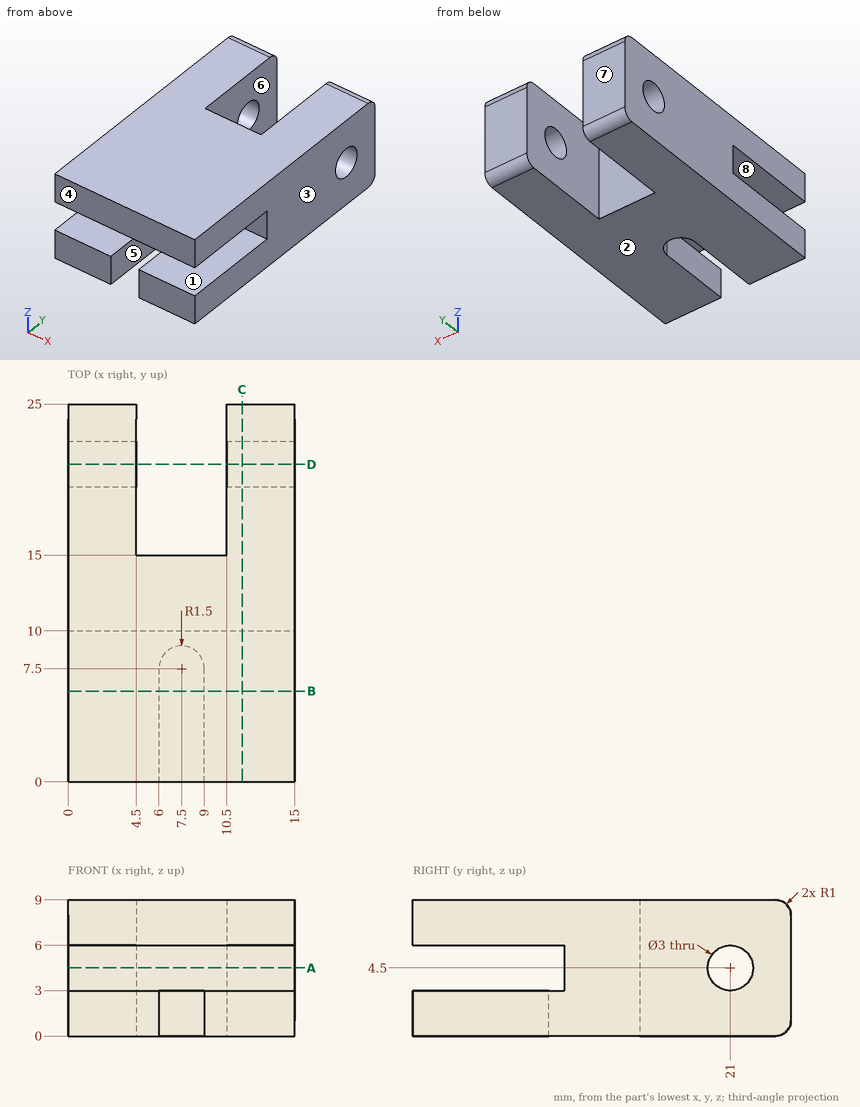
Geometry: see drawing. Coordinates: mm, zero at the bounding-box minimum. A direction names the side the tool comes from. Coordinates: 2 decimals unless noted, no trailing zeros. Loops run counter-clockwise (first coordinate to the right, second up) from the corner with the lowest first, then second, coordinate; pieces in that order, holes last. Notation, with made-up numbers: M 46.25,-35 L 103.25,-35 A31 ccw 103.25,-6 Z; hole C 18,30 d10. An arc over 180 degrees is marked long. Put each result on its own line as item: value. Start each with the question number.
1) Reachability of the marked faces 4, 5, 6, 7 and 8 from +Z, -Z, +X, -X, +Y, -Y: full face, straight path, thin tool, end or side. Return the list, or none.
2) Contact query for a flat-ended pin moving along its axis: pin 1 Ø2.5 at (x, z) = (10, 4.5) entering from -Y. Output: stop coordinate, or through.
3) Ray query, L1, parallel to X at y = 22, z = 8.25; L2, parallel to Y at x = 3.25, z = 4.5; L3, parallel to Z at x = 12.7, y = 21. Return the intervals inside material, ascending. Write a range as from..to.
4) Cut plane A-A on z = 4.5. Return the cut outline in (x, y), then the cut area to 3 significant figures.
5) Cut plane D-D on y = 21. Return the cut outline in (x, z), then the cut area to 3 significant figures.
6) Cut plane C-C on x = 11.5. Return the cut outline in (y, z), then the cut area to 3 significant figures.
7) Pull-direction query (Z, two-part tool) for the marked faces 1, 2 and 3; classes: pulls with the +Z half, pulls with the -Z half, needs draft (parallel to the pull), parting line crosses it, or undercut.
8) Cut plane B-B on y = 6. Return the cut outline in (x, z).
The answers:
1. face 4: +Z, -Z, +X, -X, -Y
1. face 5: -Z, -Y
1. face 6: +Z, -Z, +Y
1. face 7: +Z, -Z, +X, -X, +Y
1. face 8: +X, -X, -Y
2. pin 1: stops at y = 10
3. L1: x = 0..4.5, 10.5..15
3. L2: y = 10..19.5, 22.5..25
3. L3: z = 0..3, 6..9
4. outline: M 0,10 L 15,10 L 15,19.5 L 10.5,19.5 L 10.5,15 L 4.5,15 L 4.5,19.5 L 0,19.5 Z; M 0,22.5 L 4.5,22.5 L 4.5,25 L 0,25 Z; M 10.5,22.5 L 15,22.5 L 15,25 L 10.5,25 Z
4. area: 138 mm²
5. outline: M 0,0 L 4.5,0 L 4.5,3 L 0,3 Z; M 0,6 L 4.5,6 L 4.5,9 L 0,9 Z; M 10.5,0 L 15,0 L 15,3 L 10.5,3 Z; M 10.5,6 L 15,6 L 15,9 L 10.5,9 Z
5. area: 54.0 mm²
6. outline: M 0,0 L 24,0 A1 ccw 25,1 L 25,8 A1 ccw 24,9 L 0,9 L 0,6 L 10,6 L 10,3 L 0,3 Z; hole C 21,4.5 d3
6. area: 188 mm²
7. face 1: undercut
7. face 2: pulls with the -Z half
7. face 3: needs draft
8. outline: M 0,0 L 6,0 L 6,3 L 0,3 Z; M 0,6 L 15,6 L 15,9 L 0,9 Z; M 9,0 L 15,0 L 15,3 L 9,3 Z
